from build123d import *

# Parameters (mm, degrees)
BOSS_EXTRUDE1_DEPTH = 3.81
SKETCH2_R           = 1.65
CUT_EXTRUDE1_DEPTH  = 2


with BuildPart() as part:
    # Sketch1 → Boss-Extrude1 (new body, symmetric)
    with BuildSketch(Plane.XY):
        Polygon((9.55, 0), (-9.55, 0), (-9.55, -18.1), (-17.17, -18.1), (-17.17, -20.1), (-7.55, -20.1), (-7.55, -2), (7.55, -2), (7.55, -20.1), (17.17, -20.1), (17.17, -18.1), (9.55, -18.1), align=None)
    extrude(amount=BOSS_EXTRUDE1_DEPTH, both=True)

    # Sketch2 → Cut-Extrude1 (cut)
    with BuildSketch(Plane(origin=(0, -18.1, 0), x_dir=(1, 0, 0), z_dir=(0, 1, 0))):
        with Locations((-13.36, 0)):
            Circle(SKETCH2_R)
    cut_extrude1 = extrude(amount=-CUT_EXTRUDE1_DEPTH, mode=Mode.SUBTRACT)

    # Mirror1: Cut-Extrude1 across plane
    add(cut_extrude1.mirror(Plane(origin=(0, 0, 0), x_dir=(0, 0, 1), z_dir=(1, 0, 0))), mode=Mode.SUBTRACT)


solid = part.part
CAD build for the part. Positions are in the model's coordinates, mm. A direction names the side the tool comes from. Coordinates: 2 decimals unless noted, no trailing zeros. Loops run counter-clockwise (first coordinate to the right, second up) from the corner with the lowest first, then second, coordinate; pieces in that order, holes last. Notation, with made-up numbers: (51, 48) - (73, 48) arc R31 cw to (73, 79) - close; hole circle Ø10 at (70.5, 19.5). An arc over 180 degrees is marked (long way). Use one line per item in the form item = value. Start each with the question number.
1) Band-saw the part on C-C (x = 14.5). Give the cut face in (y, z), and give its area (3 significant figures).
2) Flat gauge pins, fed straight in: pin 1 (5 mm diameter, centred on x = 0.5, y = -4, fed in from +Z); pin 2 (4 mm diameter, centred on y = -10.5, z = -1.5, fed in from -X); pin 3 (2.5 mm diameter, centred on x = -12.5, z = 1.5, fed in from +Y); pin 4 (4 mm diameter, centred on x = -5, z = 0, fed in from -Y). Where does each tip first touch, or does it go through?
3) Drill centre lines: L1, parallel to X at y = -18.65, z = 0; L2, parallel to X at y = -12.5, z = 2; L3, parallel to Z at x = -13.36, y = -19. Where is each one in solid material? Low to high. Write a range as from..to.
4) Band-saw the part on D-D (z = -3). Give the cut face in (x, y).
5) Band-saw the part on A-A (z = 0). Give the cut face in (x, y).
6) Two-plate mould, pull along X, no slides. Class faces 1 (the face through (-9.55, -9, 0)), 2 (the face through (-11.836, -19.086, 0.632)), 3 (the face through (-8, -11, 3.81)): +X half, -X half, draft (parallel to the pull), parting line (faces both ways), or undercut.
7) Band-saw the part on B-B (y = -5.25). Give the cut face in (x, z).
8) Tool access for faces 4 (the face through (-13, -18.1, 2)), 5 (the face through (13, -18.1, 2)), 6 (the face through (0, -2, 0)), 7 (the face through (-11, -20.1, 0)): list every direction of +Z, -Z, +X, -X, +Y, -Y with a clear straight run to the whole face (end or side of a thin tool).
Check values:
q1.outline = (-20.1, -3.81) - (-18.1, -3.81) - (-18.1, -1.19) - (-20.1, -1.19) - close; (-20.1, 1.19) - (-18.1, 1.19) - (-18.1, 3.81) - (-20.1, 3.81) - close
q1.area = 10.5 mm2
q2.pin_1 = 3.81
q2.pin_2 = -9.55
q2.pin_3 = -18.1
q2.pin_4 = -2
q3.L1 = -17.17..-15.01, -11.71..-7.55, 7.55..11.71, 15.01..17.17
q3.L2 = -9.55..-7.55, 7.55..9.55
q3.L3 = -3.81..-1.65, 1.65..3.81
q4.outline = (-17.17, -20.1) - (-7.55, -20.1) - (-7.55, -2) - (7.55, -2) - (7.55, -20.1) - (17.17, -20.1) - (17.17, -18.1) - (9.55, -18.1) - (9.55, 0) - (-9.55, 0) - (-9.55, -18.1) - (-17.17, -18.1) - close
q5.outline = (-17.17, -20.1) - (-15.01, -20.1) - (-15.01, -18.1) - (-17.17, -18.1) - close; (-11.71, -20.1) - (-7.55, -20.1) - (-7.55, -2) - (7.55, -2) - (7.55, -20.1) - (11.71, -20.1) - (11.71, -18.1) - (9.55, -18.1) - (9.55, 0) - (-9.55, 0) - (-9.55, -18.1) - (-11.71, -18.1) - close; (15.01, -20.1) - (17.17, -20.1) - (17.17, -18.1) - (15.01, -18.1) - close
q6.face_1 = -X half
q6.face_2 = undercut
q6.face_3 = draft
q7.outline = (-9.55, -3.81) - (-7.55, -3.81) - (-7.55, 3.81) - (-9.55, 3.81) - close; (7.55, -3.81) - (9.55, -3.81) - (9.55, 3.81) - (7.55, 3.81) - close
q8.face_4 = +Z, -Z, -X, +Y
q8.face_5 = +Z, -Z, +X, +Y
q8.face_6 = +Z, -Z, -Y
q8.face_7 = +Z, -Z, +X, -X, -Y
